Design review of the part built by this model. Coordinates are the model's own, in mm. Face numbers are marked on the shaded views. A direction names the side the tool comes from. Give positions to 0.01 mm unless a question says otherwise; leave off trailing zeros. Order: outer loops, then holes, each group sorted by start corner. A loop starts at its lowest first (then second) coordinate and runs counter-clockwise, first axis right, second up.
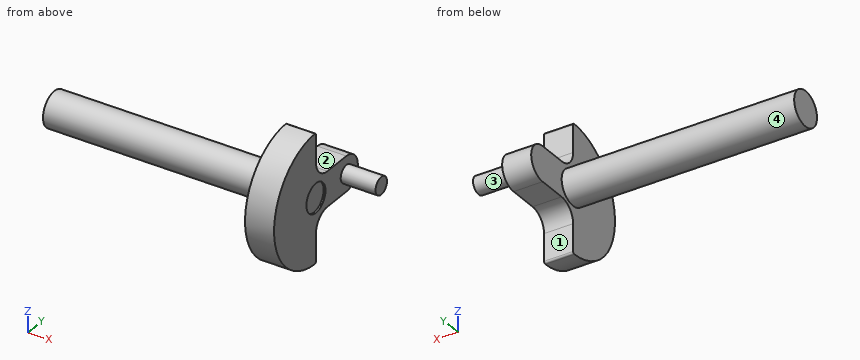
```python
from build123d import *

# Parameters (mm, degrees)
BOSS_EXTRUDE1_DEPTH = 3.96875
SKETCH4_R           = 2.38125
BOSS_EXTRUDE2_DEPTH = 31.75
SKETCH4_3_R         = 1.190625
BOSS_EXTRUDE3_DEPTH = 8.73125
SKETCH5_R           = 1.984375
CUT_EXTRUDE1_DEPTH  = 0.254


with BuildPart() as part:
    # Sketch3 → Boss-Extrude1 (new body)
    with BuildSketch(Plane(origin=(0, 0, 0), x_dir=(0, 0, -1), z_dir=(1, 0, 0))):
        with BuildLine():
            Line((-2.38125, 6.35), (-2.38125, 2.38125))
            ThreePointArc((-2.38125, 2.38125), (-3.078701977, 0.697451977), (-4.7625, 0))
            Line((-4.7625, 0), (-8.473443902, 0))
            ThreePointArc((-8.473443902, 0), (-8.655719879, -0.077106054), (-8.727329862, -0.261610487))
            ThreePointArc((-8.727329862, -0.261610487), (0, -8.73125), (8.727329862, -0.261610487))
            ThreePointArc((8.727329862, -0.261610487), (8.655719879, -0.077106054), (8.473443902, 0))
            Line((8.473443902, 0), (4.7625, 0))
            ThreePointArc((4.7625, 0), (3.078701977, 0.697451977), (2.38125, 2.38125))
            Line((2.38125, 2.38125), (2.38125, 6.35))
            ThreePointArc((2.38125, 6.35), (0, 8.73125), (-2.38125, 6.35))
        make_face()
    extrude(amount=BOSS_EXTRUDE1_DEPTH)

    # Sketch4 → Boss-Extrude2 (add)
    with BuildSketch(Plane.ZY):
        Circle(SKETCH4_R)
    extrude(amount=BOSS_EXTRUDE2_DEPTH)

    # Sketch4<3> → Boss-Extrude3 (add)
    with BuildSketch(Plane.ZY):
        with Locations((0, 6.35)):
            Circle(SKETCH4_3_R)
    extrude(amount=-BOSS_EXTRUDE3_DEPTH)

    # Sketch5 → Cut-Extrude1 (cut)
    with BuildSketch(Plane(origin=(3.96875, 0, 0), x_dir=(0, 0, -1), z_dir=(1, 0, 0))):
        Circle(SKETCH5_R)
    extrude(amount=-CUT_EXTRUDE1_DEPTH, mode=Mode.SUBTRACT)


solid = part.part
```
1. Machinability: for the marked faces 1, 2, 3 and 4, which of the approach directions +Z, -Z, +X, -X, +Y, -Y give a long, thin tool a straight path to every point of the face, cutting with its end or side? Answer none if there is none.
Recorded:
face 1: -Z, +X, -X, +Y
face 2: +Z, +X, -X, +Y
face 3: +X
face 4: -X
2. Take a section at A-A (z = 0). State the section outline as (x, y) points, then the cut area to 3 significant figures.
Recorded:
outline: (-31.75, -2.38) - (0, -2.38) - (0, -8.73) - (3.97, -8.73) - (3.97, -1.98) - (3.71, -1.98) - (3.71, 1.98) - (3.97, 1.98) - (3.97, 5.16) - (8.73, 5.16) - (8.73, 7.54) - (3.97, 7.54) - (3.97, 8.73) - (0, 8.73) - (0, 2.38) - (-31.75, 2.38) - close
area: 231 mm2
3. For pin 1 (1.5 mm diameter, centred on x = -4, z = 2, fed in from -Y); pin 2 (1.2 mm diameter, centred on x = 1.5, y = 4.5, fed in from +Z); pin 3 (2 mm diameter, centred on x = 2.5, y = 5, fed in from -Z); pin 4 (8 mm diameter, centred on y = 4.5, z = -3, fed in from +X), all flat-tipped, find the tip position at first contact; note any pin that passes through.
Recorded:
pin 1: stops at y = -2.03
pin 2: stops at z = 2.38
pin 3: stops at z = -2.38
pin 4: stops at x = 8.73
4. Take a section at D-D (z = -7.25). State the section outline as (x, y) points, then the cut area to 3 significant figures.
Recorded:
outline: (0, -4.87) - (3.97, -4.87) - (3.97, 0) - (0, 0) - close
area: 19.3 mm2
5. Take a section at B-B (x = -8.5). State the section outline as (y, z) points.
Recorded:
outline: circle Ø4.76 at (0, 0)
6. For line 1 along Y through (x, z) = (3.8, 0); line 2 along X through (y, z) = (-6.75, 0.75); line 3 along X through (y, z) = (-2.25, 0), list the stretches that pass through material, from the lowest coordinate up.
Recorded:
line 1: y = -8.73 to -1.98, 1.98 to 8.73
line 2: x = 0 to 3.97
line 3: x = -31.75 to 3.97
7. Take a section at C-C (y = -6.75). State the section outline as (x, z) points.
Recorded:
outline: (0, -5.54) - (3.97, -5.54) - (3.97, 5.54) - (0, 5.54) - close
